```python
from build123d import *

# Parameters (mm, degrees)
SKETCH4_W           = 32
SKETCH4_H           = 16
BOSS_EXTRUDE3_DEPTH = 1.6
SKETCH5_W           = 32
SKETCH5_H           = 2.4
BOSS_EXTRUDE4_DEPTH = 6
SKETCH6_W           = 32
SKETCH6_H           = 7.6
SKETCH6_W_2         = 30.4
SKETCH6_H_2         = 6
BOSS_EXTRUDE5_DEPTH = 4.8
SKETCH7_W           = 12
SKETCH7_H           = 0.8
CUT_EXTRUDE1_DEPTH  = 4.8
SKETCH8_W           = 26
SKETCH8_H           = 0.8
BOSS_EXTRUDE6_DEPTH = 12
SKETCH9_W           = 0.8
SKETCH9_H           = 12.8
BOSS_EXTRUDE7_DEPTH = 4.8
SKETCH10_W          = 74.676808058
SKETCH10_H          = 45.618872406
CUT_EXTRUDE2_DEPTH  = 5.6
FILLET1_R           = 2


with BuildPart() as part:
    # Sketch4 → Boss-Extrude3 (new body)
    with BuildSketch(Plane.XY):
        with Locations((16, -8)):
            Rectangle(SKETCH4_W, SKETCH4_H)
    extrude(amount=BOSS_EXTRUDE3_DEPTH)

    # Sketch5 → Boss-Extrude4 (add)
    with BuildSketch(Plane(origin=(0, 0, 0), x_dir=(-1, 0, 0), z_dir=(0, 0, -1))):
        with Locations((-16, -1.2)):
            Rectangle(SKETCH5_W, SKETCH5_H)
    extrude(amount=BOSS_EXTRUDE4_DEPTH)

    # Sketch6 → Boss-Extrude5 (add)
    with BuildSketch(Plane(origin=(0, 0, 0), x_dir=(1, 0, 0), z_dir=(0, 1, 0))):
        with Locations((16, 2.2)):
            Rectangle(SKETCH6_W, SKETCH6_H)
        with Locations((16, 2.2)):
            Rectangle(SKETCH6_W_2, SKETCH6_H_2, mode=Mode.SUBTRACT)
    extrude(amount=BOSS_EXTRUDE5_DEPTH)

    # Sketch7 → Cut-Extrude1 (cut)
    with BuildSketch(Plane(origin=(0, 4.8, 0), x_dir=(1, 0, 0), z_dir=(0, 1, 0))):
        with Locations((16, -1.2)):
            Rectangle(SKETCH7_W, SKETCH7_H)
    extrude(amount=-CUT_EXTRUDE1_DEPTH, mode=Mode.SUBTRACT)

    # Sketch8 → Boss-Extrude6 (add)
    with BuildSketch(Plane.XY.offset(1.6)):
        with Locations((23, -0.4)):
            Rectangle(SKETCH8_W, SKETCH8_H)
    extrude(amount=BOSS_EXTRUDE6_DEPTH)

    # Sketch9 → Boss-Extrude7 (add)
    with BuildSketch(Plane(origin=(0, 0, 0), x_dir=(1, 0, 0), z_dir=(0, 1, 0))):
        with Locations((10.4, -7.2)):
            Rectangle(SKETCH9_W, SKETCH9_H)
        with Locations((35.6, -7.2)):
            Rectangle(SKETCH9_W, SKETCH9_H)
    extrude(amount=BOSS_EXTRUDE7_DEPTH)

    # Sketch10 → Cut-Extrude2 (cut)
    with BuildSketch(Plane(origin=(0, 4.8, 0), x_dir=(1, 0, 0), z_dir=(0, 1, 0))):
        with Locations((31.433625096, -2.501503002)):
            Rectangle(SKETCH10_W, SKETCH10_H)
    extrude(amount=-CUT_EXTRUDE2_DEPTH, mode=Mode.SUBTRACT)

    # Fillet1
    fillet1_edges = [part.edges().sort_by_distance(p)[0] for p in [
        (16, -2.4, 0),
    ]]
    fillet(fillet1_edges, radius=FILLET1_R)


solid = part.part
```
Read the model definition and answer for the solid it produces. Units are mm, in the model's axes. A direction names the side the tool comes from. Give positions to 0.01 mm unless a question says otherwise; leave off trailing zeros. Order: outer loops, then holes, each group sorted by start corner. A loop starts at its lowest first (then second) coordinate and runs counter-clockwise, first axis right, second up.
(1) Straight lines are drawn through the part: L1, parallel to Z at x = 16, y = -8.5; L2, parallel to Y at x = 28, z = -3.25; L3, parallel to Y at x = 28, z = -0.25. For each, find the intervals that lie inside material, in ascending order.
(2) Given pin 1 (3 mm diameter, centred on x = 18, z = -3.5, fed in from -Y); pin 2 (6 mm diameter, centred on x = 14.5, y = -14, fed in from -Z), each flat-ended and moving along its own axis, determine where each tip first touches the part or whether it passes through.
(3) For faces 1 (the flat face through (16, -16, 1)), 2 (the flat face through (16, -2.4, -4)), determine the directions among +Z, -Z, +X, -X, +Y, -Y from which every point of the face is accessible in a straight line to the end or side of a thin tool.
(4) Find section A-A (x = 19). Give the vertices of the cut face in (y, z), plus the area to 3 significant figures.
(5) Find section B-B (z = -4.5). Give the vertices of the cut face in (x, y).
(6) Find section C-C (y = -6.75). Give the vertices of the cut face in (x, z), plus the area to 3 significant figures.
Result sheet:
1. L1: z = 0 to 1.6
1. L2: y = -2.4 to -0.8
1. L3: y = -3.43 to -0.8
2. pin 1: stops at y = -2.4
2. pin 2: stops at z = 0
3. face 1: +Z, -Z, +X, -X, -Y
3. face 2: -Z, +X, -X, -Y
4. outline: (-16, 0) - (-4.4, 0) arc R2 cw to (-2.4, -2) - (-2.4, -6) - (-0.8, -6) - (-0.8, 1.6) - (-16, 1.6) - close
4. area: 34.8 mm2
5. outline: (0, -2.4) - (32, -2.4) - (32, -0.8) - (0, -0.8) - close
6. outline: (0, 0) - (32, 0) - (32, 1.6) - (0, 1.6) - close
6. area: 51.2 mm2
